Could you check a few things on this model? Use its own coordinates, in mm. A direction names the side the tool comes from. Coordinates: 2 decimals unless noted, no trailing zeros. Write each loop counter-clockwise with the first axis right and the second up, starting at its lowest first coordinate (ties: lowest second). Pieces come first, ordered by that corner, then holes. Notation, with made-up numbers: (-13, 67.25) - (0, 67.25) arc R15 cw to (0, 81.25) - close; hole circle Ø2 at (-24, 34). An arc over 180 degrees is marked (long way). Write item = value, one per line. Start each with the question number.
```python
from build123d import *

# Parameters (mm, degrees)
BOSS_EXTRUDE1_DEPTH = 18
CUT_EXTRUDE1_DEPTH  = 7
BOSS_EXTRUDE2_DEPTH = 7
SKETCH4_R           = 2.5
CUT_EXTRUDE2_DEPTH  = 6
SKETCH5_R           = 5.75
CUT_EXTRUDE3_DEPTH  = 7
CUT_EXTRUDE4_START  = -7
SKETCH6_R           = 5.75
CUT_EXTRUDE4_DEPTH  = 7
SCALE1_SCALE        = 0.75
SCALE2_SCALE        = 1.066666667


with BuildPart() as part:
    # Sketch1 → Boss-Extrude1 (new body)
    with BuildSketch(Plane(origin=(0, 0, 0), x_dir=(1, 0, 0), z_dir=(0, 1, 0))):
        with BuildLine():
            Line((10.653013329, -29.309744988), (10.653013329, -30.57769418))
            ThreePointArc((10.653013329, -30.57769418), (11.653013329, -34.309744988), (12.653013329, -30.57769418))
            Line((12.653013329, -30.57769418), (12.653013329, -29.309744988))
            Line((12.653013329, -29.309744988), (14.653013329, -29.309744988))
            Line((14.653013329, -29.309744988), (17.5, -26.5))
            Line((17.5, -26.5), (22.5, -26.5))
            Line((22.5, -26.5), (22.5, 26.5))
            Line((22.5, 26.5), (16.5, 26.5))
            Line((16.5, 26.5), (12.844502727, 30.107679392))
            Line((12.844502727, 30.107679392), (11.410696035, 30.107679392))
            ThreePointArc((11.410696035, 30.107679392), (11.225950376, 29.984289062), (11.269162996, 29.766369807))
            ThreePointArc((11.269162996, 29.766369807), (9.5, 25.5), (7.730837004, 29.766369807))
            ThreePointArc((7.730837004, 29.766369807), (7.774049624, 29.984289062), (7.589303965, 30.107679392))
            Line((7.589303965, 30.107679392), (6.155497273, 30.107679392))
            Line((6.155497273, 30.107679392), (2.5, 26.5))
            Line((2.5, 26.5), (-9.870833143, 26.5))
            ThreePointArc((-9.870833143, 26.5), (-10.486603861, 26.436124388), (-11.076152757, 26.247217616))
            Line((-11.076152757, 26.247217616), (-20.702456422, 22.023754373))
            Line((-20.702456422, 22.023754373), (-20.705319614, 22.022498171))
            ThreePointArc((-20.705319614, 22.022498171), (-22.011569115, 20.916018371), (-22.5, 19.275280555))
            Line((-22.5, 19.275280555), (-22.5, 17.88854382))
            ThreePointArc((-22.5, 17.88854382), (-21.987950036, 17.015672259), (-20.976190476, 17.0367084))
            ThreePointArc((-20.976190476, 17.0367084), (9.5, 0), (-20.976190476, -17.0367084))
            ThreePointArc((-20.976190476, -17.0367084), (-21.987950036, -17.015672259), (-22.5, -17.88854382))
            Line((-22.5, -17.88854382), (-22.5, -19.287953276))
            ThreePointArc((-22.5, -19.287953276), (-22.010713993, -20.929999331), (-20.702456502, -22.03642528))
            Line((-20.702456502, -22.03642528), (-11.074921132, -26.248472005))
            ThreePointArc((-11.074921132, -26.248472005), (-10.486705619, -26.43644479), (-9.87246463, -26.5))
            Line((-9.87246463, -26.5), (5.880022863, -26.5))
            Line((5.880022863, -26.5), (8.653013329, -29.309744988))
            Line((8.653013329, -29.309744988), (10.653013329, -29.309744988))
        make_face()
    extrude(amount=BOSS_EXTRUDE1_DEPTH)

    # Sketch2 → Cut-Extrude1 (cut)
    with BuildSketch(Plane.XZ):
        with BuildLine():
            Line((18.5, 22.5), (18.5, -22.5))
            Line((18.5, -22.5), (-2.148353456, -22.5))
            ThreePointArc((-2.148353456, -22.5), (13.5, 0), (-2.148353456, 22.5))
            Line((-2.148353456, 22.5), (7.238559187, 22.5))
            Line((7.238559187, 22.5), (10.039345887, 25.282038261))
            Line((10.039345887, 25.282038261), (13.039345883, 25.282178795))
            Line((13.039345883, 25.282178795), (15.843268341, 22.5))
            Line((15.843268341, 22.5), (18.5, 22.5))
        make_face()
    cut_extrude1 = extrude(amount=-CUT_EXTRUDE1_DEPTH, mode=Mode.SUBTRACT)

    # Mirror1: Cut-Extrude1 across plane
    add(cut_extrude1.mirror(Plane(origin=(0, 9, 0), x_dir=(0, 0, 1), z_dir=(0, -1, 0))), mode=Mode.SUBTRACT)

    # Sketch3 → Boss-Extrude2 (add)
    with BuildSketch(Plane.ZY.offset(-18.5)):
        with BuildLine():
            Line((7, 7), (-7, 7))
            ThreePointArc((-7, 7), (0, 0), (7, 7))
        make_face()
    boss_extrude2 = extrude(amount=BOSS_EXTRUDE2_DEPTH)

    # Mirror2: Boss-Extrude2 across plane
    add(boss_extrude2.mirror(Plane(origin=(0, 9, 0), x_dir=(0, 0, 1), z_dir=(0, -1, 0))))

    # Sketch4 → Cut-Extrude2 (cut)
    with BuildSketch(Plane(origin=(22.5, 0, 0), x_dir=(0, 0, -1), z_dir=(1, 0, 0))):
        with Locations((0, 9)):
            Circle(SKETCH4_R)
    extrude(amount=-CUT_EXTRUDE2_DEPTH, mode=Mode.SUBTRACT)

    # Sketch5 → Cut-Extrude3 (cut)
    with BuildSketch(Plane(origin=(9.5, 0, 0), x_dir=(0, 0, -1), z_dir=(1, 0, 0))):
        with Locations((0, 9)):
            Circle(SKETCH5_R)
    extrude(amount=-CUT_EXTRUDE3_DEPTH, mode=Mode.SUBTRACT)

    # Sketch6 → Cut-Extrude4 (cut)
    with BuildSketch(Plane.ZY.offset(-9.5).offset(CUT_EXTRUDE4_START)):
        with Locations(Location((0, 9, 0), (0, 0, 180))):
            Circle(SKETCH6_R)
    extrude(amount=CUT_EXTRUDE4_DEPTH, mode=Mode.SUBTRACT)


with BuildPart() as part_1:
    # Scale1: scaled about (0, 0, 0)
    add(part.part.scale(SCALE1_SCALE))


with BuildPart() as part_2:
    # Scale2: scaled about (0, 0, 0)
    add(part_1.part.scale(SCALE2_SCALE))


solid = part_2.part
```
1) Suppose I cut it at C-C on z = -8. Please give me the cut outline in (x, y), plus the area to 3 significant figures.
2) Suppose I cut it at D-D on x = -13.5. Please give me the cut outline in (y, z).
3) Suppose I cut it at A-A on x = 3. Please give me the cut outline in (y, z), plus the area to 3 significant figures.
4) For P1, Ø3, axis at y = 10.5, z = -8.5, coming from the -X side; P2, Ø1.5, axis at x = 1, y = 5, coming from the -Z side; P3, Ø1.7, axis at x = 2, y = 13, coming from the -Z side, each with a flat end and sliding along its axis, tell me the tip position at first contact or that it passes through.
5) If I drill on probe 1 along Z at (x, y) = (13, 2.25); probe 2 along Z at (x, y) = (1.5, 5.25); probe 3 along Z at (x, y) = (4, 10.5), over which ranges is the centre line in solid material (lowest first)? Write a range as [from, to].
6) Suppose I cut it at B-B on z = -22.4. Please give me the cut outline in (x, y), plus the area to 3 significant figures.
7) Thinking about a two-plate mould opening in Z: for faces 1 (the flat face through (18, 4, 0)), 2 (the flat face through (16, 7, -21.2)), 3 (the flat face through (10, 5.6, -13)), which applies, +Z half, -Z half, draft (parallel to the pull), parting line (faces both ways), or undercut?
8) Which directions (+Z, -Z, +X, -X, +Y, -Y) give clear straight access to the entire face, cutting with the end or side of a thin tool? Please do faces 4 (the flat face through (5.5, 7.1, -24.086)), 5 (the cylindrical face through (12.4, 14.4, -0.1)), 6 (the flat face through (14.8, 3, -11)).
Reply:
q1.outline = (5.46, 0) - (9.05, 0) - (9.05, 5.6) - (14.8, 5.6) - (14.8, 0) - (18, 0) - (18, 14.4) - (14.8, 14.4) - (14.8, 8.8) - (9.05, 8.8) - (9.05, 14.4) - (5.46, 14.4) - close
q1.area = 116 mm^2
q2.outline = (0, -18.96) - (14.4, -18.96) - (14.4, -15.17) - (0, -15.17) - close; (0, 15.17) - (14.4, 15.17) - (14.4, 18.97) - (0, 18.97) - close
q3.outline = (0, -22.19) - (14.4, -22.19) - (14.4, -18) - (8.8, -18) - (8.8, -15.45) - (14.4, -15.45) - (14.4, -11.23) - (0, -11.23) - (0, -15.45) - (5.6, -15.45) - (5.6, -18) - (0, -18) - close; (0, 11.23) - (14.4, 11.23) - (14.4, 15.45) - (8.8, 15.45) - (8.8, 18) - (14.4, 18) - (14.4, 21.2) - (0, 21.2) - (0, 18) - (5.6, 18) - (5.6, 15.45) - (0, 15.45) - close
q3.area = 244 mm^2
q4.P1 = 4.09
q4.P2 = -21.2
q4.P3 = -22.04
q5.probe_1 = [-21.4, -18], [-4.49, 4.49], [18, 22.19]
q5.probe_2 = [-21.2, -18], [-16.45, -12.57], [12.57, 16.45], [18, 21.2]
q5.probe_3 = [-23.17, -18], [-14.66, -10.11], [10.11, 14.66], [18, 21.2]
q6.outline = (3.22, 0) - (5.6, 0) - (5.6, 14.4) - (3.22, 14.4) - close; (9.6, 0) - (11.98, 0) - (11.98, 14.4) - (9.6, 14.4) - close
q6.area = 68.7 mm^2
q7.face_1 = draft
q7.face_2 = -Z half
q7.face_3 = undercut
q8.face_4 = -Z, +X, -X, +Y, -Y
q8.face_5 = +Y
q8.face_6 = -Y
